Here's how the part is built. I have some questions about the finished solid (model axes, mm). Round coordinates to 2 decimals unless told otherwise and drop trailing zeros. Write each loop counter-clockwise with the first axis right and the second up, starting at its lowest first coordinate (ties: lowest second). Pieces come first, ordered by that corner, then holes. Notation, with made-up numbers: (27.25, 84.5) -> (63.25, 84.5) arc R30 ccw to (63.25, 114.5) -> close; hole circle Ø4 at (11.25, 89.25). An arc over 180 degrees is marked (long way). Put each result on its own line as item: value. Start each with the question number.
1) I want a section at B-B, the plane x = -5. List the corners of the cut face in (y, z) for me, then the cut area to 3 significant figures.
2) I want a section at C-C, the plane z = 2.4. List the corners of the cut face in (x, y) for me.
3) Will these pins go through, and if not, where does the flat tip stop? P1, Ø4.5, axis at x = -17.96, y = 17.96, coming from the +Z side; P2, Ø15, axis at x = 0, y = 0, coming from the +Z side; P3, Ø3, axis at x = 1.5, z = 1.5, coming from the +Y side.
4) We'd pull the mould along X, two halves only. Please class faces 1 (the flat face through (30, -32, 2)), 2 (the cylindrical face through (-0.66, 29.993, 2.465)), 3 (the cylindrical face through (-19.547, 16.743, 2.465)), 4 (the flat face through (-30, -33, 2)): released by +X, released by -X, zero draft, split by the parting line, or undercut.
5) I want a section at A-A, the plane y = -17.96. List the corners of the cut face in (x, z) for me.
6) If I drill on line 1 along Y through (x, z) = (25.4, 3.45); line 2 along Y through (x, z) = (0, 1.8); line 3 along X through (y, z) = (3, 2.9), over which ranges is the centre line in solid material (lowest first)? Write a range as [from, to].
from build123d import *

# Parameters (mm, degrees)
SKETCH_1_R      = 2
SKETCH_1_R_2    = 12.5
EXTRUDE_1_DEPTH = 5


with BuildPart() as part:
    # 草图1 → 凸台-拉伸1 (new body)
    with BuildSketch(Plane.XY):
        with BuildLine():
            Line((30, -65), (-30, -65))
            Line((-30, -65), (-30, 0))
            ThreePointArc((-30, 0), (0, 30), (30, 0))
            Line((30, 0), (30, -65))
        make_face()
        with Locations((-17.96, 17.96)):
            Circle(SKETCH_1_R, mode=Mode.SUBTRACT)
        with Locations((-25.4, 0)):
            Circle(SKETCH_1_R, mode=Mode.SUBTRACT)
        with Locations(Location((25.4, 0, 0), (0, 0, 180))):
            Circle(SKETCH_1_R, mode=Mode.SUBTRACT)
        with Locations((17.96, -17.96)):
            Circle(SKETCH_1_R, mode=Mode.SUBTRACT)
        Circle(SKETCH_1_R_2, mode=Mode.SUBTRACT)
    extrude(amount=EXTRUDE_1_DEPTH)


solid = part.part
Findings:
1. outline: (-65, 0) -> (-11.46, 0) -> (-11.46, 5) -> (-65, 5) -> close; (11.46, 0) -> (29.58, 0) -> (29.58, 5) -> (11.46, 5) -> close
1. area: 358 mm2
2. outline: (-30, -65) -> (30, -65) -> (30, 0) arc R30 ccw to (-30, 0) -> close; hole circle Ø4 at (-25.4, 0); hole circle Ø4 at (-17.96, 17.96); hole circle Ø25 at (0, 0); hole circle Ø4 at (17.96, -17.96); hole circle Ø4 at (25.4, 0)
3. P1: stops at z = 5
3. P2: passes through
3. P3: stops at y = 30
4. face 1: released by +X
4. face 2: split by the parting line
4. face 3: undercut
4. face 4: released by -X
5. outline: (-30, 0) -> (15.96, 0) -> (15.96, 5) -> (-30, 5) -> close; (19.96, 0) -> (30, 0) -> (30, 5) -> (19.96, 5) -> close
6. line 1: y = [-65, -2], [2, 15.96]
6. line 2: y = [-65, -12.5], [12.5, 30]
6. line 3: x = [-29.85, -12.13], [12.13, 29.85]
